Autodesk Inventor part; units mm, degrees
ref_plane "YZ Plane" through (0, 0, 0) normal (1, 0, 0) x (0, 1, 0)
ref_plane "XZ Plane" through (0, 0, 0) normal (0, 1, 0) x (-1, 0, 0)
ref_plane "XY Plane" through (0, 0, 0) normal (0, 0, 1) x (1, 0, 0)
sketch "Skizze1" plane through (0, 0, 0) normal (0, 0, 1) x (1, 0, 0)
  line L0 (-10, -5) -> (10, -5)
  line L1 (10, -5) -> (10, 5)
  line L2 (10, 5) -> (-10, 5)
  line L3 (-10, 5) -> (-10, -5)
  line L4 (-10, -5) -> (10, 5) construction
  line L5 (10, -5) -> (-10, 5) construction
  circle A0 centre (0, 0) radius 2
  circle A1 centre (-6.5, 0) radius 2
  circle A2 centre (6.5, 0) radius 2
  line L6 (-10, 0) -> (10, 0) construction
  dimension "d0" = 10
  dimension "d1" = 20
  dimension "d2" = 4
  dimension "d3" = 6.5
  dimension "d4" = 6.5
extrude "Extrusion1" add sketch "Skizze1" along normal blind 15 contours L3 L2 L1 L0 | A0 | A1 | A2
sketch "Skizze2" plane through (0, 0, 15) normal (0, 0, 1) x (1, 0, 0)
  point P0 (0, 0)
hole "Bohrung1" at (0, 0, 15) direction (0, 0, -1) diameter 3.242 end through all
sketch "Skizze3" plane through (0, 0, 0) normal (0, 0, -1) x (-1, 0, 0)
  point P0 (0, 0)
  point P1 (-6.5, 0)
  point P2 (6.5, 0)
hole "Bohrung2" at (6.5, 0, 0) at (-6.5, 0, 0) direction (0, 0, 1) diameter 3.242 end through all
properties part number "Alu_Belt_tens" material "Aluminium 6061"
Part model, mm, in its own coordinate system. Coordinates: 2 decimals unless noted, no trailing zeros. Order: outer loops, then holes, each group sorted by start corner. A loop starts at its lowest first (then second) coordinate and runs counter-clockwise, first axis right, second up. Notation, with made-up numbers: M 3,12 L 34,12 A13 cw 34,17 Z; hole C -9,30.5 d1. An arc over 180 degrees is marked long. One line per question, with ' | ' between items.
Q1. Drill centre lines: line 1 (X direction, y = 0, z = 5.5); line 2 (Y direction, x = 6.5, z = 9); line 3 (Y direction, x = -0.5, z = 5). Where is each one in solid material? Low to high.
A:
line 1: x = -10 to -8.12, -4.88 to -1.62, 1.62 to 4.88, 8.12 to 10 | line 2: y = -5 to -1.62, 1.62 to 5 | line 3: y = -5 to -1.54, 1.54 to 5
Q2. Two-plate mould, pull along X, no slides. Class faces 1 (the face through (5.13, 0.87, 7.6)), 2 (the face through (-5.062, 0.748, 7.605)), 3 (the face through (10, 0, 7)), 4 (the face through (0, -5, 7)): +X half, -X half, draft (parallel to the pull), parting line (faces both ways), or undercut.
A:
face 1: undercut | face 2: undercut | face 3: +X half | face 4: draft
Q3. Slice it at A-A (x = -6.5). Give the cut face in (y, z), and give its area (3 significant figures).
A:
outline: M -5,0 L -1.62,0 L -1.62,15 L -5,15 Z; M 1.62,0 L 5,0 L 5,15 L 1.62,15 Z | area: 101 mm^2
Q4. Slice it at D-D (x = 1). Give the cut face in (y, z).
A:
outline: M -5,0 L -1.28,0 L -1.28,15 L -5,15 Z; M 1.28,0 L 5,0 L 5,15 L 1.28,15 Z
Q5. Slice it at B-B (z = 2.25). Give the cut face in (x, y).
A:
outline: M -10,-5 L 10,-5 L 10,5 L -10,5 Z; hole C -6.5,0 d3.24; hole C 0,0 d3.24; hole C 6.5,0 d3.24
Q6. Slice it at C-C (y = 0). Give the cut face in (x, z).
A:
outline: M -10,0 L -8.12,0 L -8.12,15 L -10,15 Z; M -4.88,0 L -1.62,0 L -1.62,15 L -4.88,15 Z; M 1.62,0 L 4.88,0 L 4.88,15 L 1.62,15 Z; M 8.12,0 L 10,0 L 10,15 L 8.12,15 Z
